from build123d import *

# Parameters (mm, degrees)
F0_R          = 24.13
F1_DEPTH      = 38.1
F2_R          = 22.86
F3_DEPTH      = 25.4
F3_DEPTH_BACK = 25.4
F5_R          = 6.35
F6_DEPTH      = 25.4
F6_DEPTH_BACK = 25.4


with BuildPart() as f1:
    # F0 (on Top) → F1 (new body)
    with BuildSketch(Plane.XY):
        Circle(F0_R)
    extrude(amount=F1_DEPTH)

    # F2 (on Right) → F3 (cut, two sides)
    with BuildSketch(Plane.YZ) as f3_sk:
        Circle(F2_R)
    extrude(amount=-F3_DEPTH, mode=Mode.SUBTRACT)
    extrude(f3_sk.sketch, amount=F3_DEPTH_BACK, mode=Mode.SUBTRACT)

    # F5 (on face) → F6 (cut, two sides)
    with BuildSketch(Plane.XZ) as f6_sk:
        with Locations((0, 14.1012268141)):
            Circle(F5_R)
    extrude(amount=-F6_DEPTH, mode=Mode.SUBTRACT)
    extrude(f6_sk.sketch, amount=F6_DEPTH_BACK, mode=Mode.SUBTRACT)


solid = f1.part
The listing builds one solid part. Answer for the finished solid, in the listing's coordinates (mm). Give positions to 0.01 mm unless a question says otherwise; leave off trailing zeros. Write each loop counter-clockwise with the first axis right and the second up, starting at its lowest first coordinate (ties: lowest second). Pieces come first, ordered by that corner, then holes.
Item 1: Section C-C, the plane y = 14 is taken. Write down the section's boundary in (x, z).
Item 2: Find the intervals of material crossed by line 1 along Z through (x, y) = (0, -16.5); line 2 along Y through (x, z) = (-15, 20); line 3 along Y through (x, z) = (-11.5, 14), in increasing order.
Item 3: Section A-A, the plane z = 18 is taken. Write down the section's boundary in (x, y).
Item 4: Flat-ended cylindrical pins translate along their axes: P1, Ø12, axis at x = -17.5, z = 7.5, coming from the +Y side; P2, Ø4, axis at y = 4, z = 26.5, coming from the -X side; P3, Ø1, axis at y = 12.5, z = 29, coming from the +X side; P4, Ø11.5, axis at x = 0, z = 14.1, coming from the -Y side. Find the tip coordinate at first contact, or state that the pin passes through.
Item 5: Determine the mould class of faces 1 (the cylindrical face through (-0.8, -18.6, 20.4)), 2 (the flat face through (0, 0, 38.1)), 3 (the cylindrical face through (-5.231, -23.556, 23.017)) for opening direction X: released by +X, released by -X, zero draft, split by the parting line, or undercut.
Item 6: Section B-B, the plane z = 22 is taken. Write down the section's boundary in (x, y).
Item 7: Section D-D, the plane x = 15.5 is taken. Write down the section's boundary in (y, z).
Completed:
1. outline: (-19.65, 18.07) - (-4.96, 18.07) arc R6.35 cw to (4.96, 18.07) - (19.65, 18.07) - (19.65, 38.1) - (-19.65, 38.1) - close
2. line 1: z = 20.45 to 38.1
2. line 2: y = -18.9 to -11.07, 11.07 to 18.9
2. line 3: y = -21.21 to -18.07, 18.07 to 21.21
3. outline: (-19.59, -14.09) arc R24.13 ccw to (-5.01, -23.6) - (-5.01, -14.09) - close; (-19.59, 14.09) - (-5.01, 14.09) - (-5.01, 23.6) arc R24.13 ccw to start; (5.01, -23.6) arc R24.13 ccw to (19.59, -14.09) - (5.01, -14.09) - close; (5.01, 14.09) - (19.59, 14.09) arc R24.13 ccw to (5.01, 23.6) - close
4. P1: stops at y = 21.15
4. P2: stops at x = -24.05
4. P3: stops at x = 20.93
4. P4: passes through
5. face 1: undercut
5. face 2: zero draft
5. face 3: split by the parting line
6. outline: (-23.32, -6.21) arc R24.13 ccw to (23.32, -6.21) - close; (-23.32, 6.21) - (23.32, 6.21) arc R24.13 ccw to start
7. outline: (-18.49, 13.44) arc R22.86 cw to (18.49, 13.44) - (18.49, 38.1) - (-18.49, 38.1) - close
